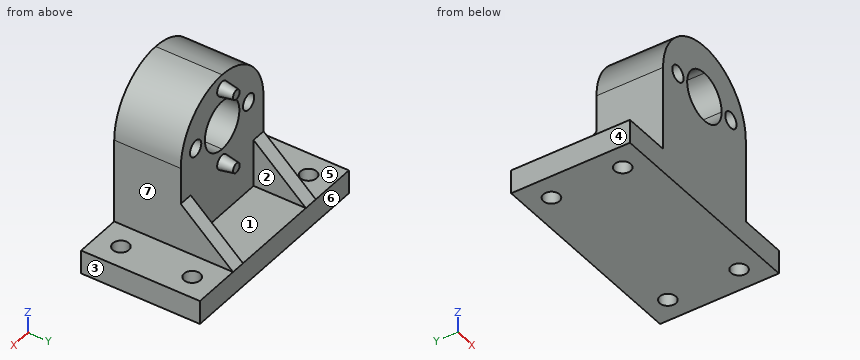
from build123d import *
from OCP.BRepFilletAPI import BRepFilletAPI_MakeChamfer

# Parameters (mm, degrees)
SKETCH1_R           = 1.7
BOSS_EXTRUDE1_DEPTH = 5
SKETCH2_R           = 1.7
BOSS_EXTRUDE2_DEPTH = 14
SKETCH3_R           = 1.5
BOSS_EXTRUDE3_DEPTH = 3
CHAMFER1_SIZE       = 3
CHAMFER1_SIZE_2     = 0.5
FILLET1_R           = 12.5
SKETCH4_W           = 3
SKETCH4_H           = 10
BOSS_EXTRUDE4_DEPTH = 11
CHAMFER2_SIZE       = 10
CHAMFER2_SIZE_2     = 11


with BuildPart() as part:
    # Sketch1 → Boss-Extrude1 (new body)
    with BuildSketch(Plane.XY):
        Polygon((-93.960167873, 235.92362241), (-129.123766163, 235.92362241), (-134.123766163, 235.92362241), (-134.123766163, 210.92362241), (-129.123766163, 210.92362241), (-93.960167873, 210.92362241), (-89.123766163, 210.92362241), (-89.123766163, 235.92362241), align=None)
        with Locations((-93.960167873, 215.92362241)):
            Circle(SKETCH1_R, mode=Mode.SUBTRACT)
        with Locations((-93.960167873, 230.92362241)):
            Circle(SKETCH1_R, mode=Mode.SUBTRACT)
        with Locations((-129.123766163, 215.92362241)):
            Circle(SKETCH1_R, mode=Mode.SUBTRACT)
        with Locations((-129.123766163, 230.92362241)):
            Circle(SKETCH1_R, mode=Mode.SUBTRACT)
    extrude(amount=BOSS_EXTRUDE1_DEPTH)

    # Sketch2 → Boss-Extrude2 (add)
    # profile 1 of 2: a face of its own
    with BuildSketch(Plane.XZ.offset(-210.92362241)):
        with BuildLine():
            Line((-111.623766166, 19.049999998), (-111.623766166, 5))
            Line((-111.623766166, 5), (-99.123766166, 5))
            Line((-99.123766166, 5), (-99.123766166, 35.249999998))
            Line((-99.123766166, 35.249999998), (-111.623766166, 35.249999998))
            Line((-111.623766166, 35.249999998), (-111.623766166, 29.449999998))
            ThreePointArc((-111.623766166, 29.449999998), (-107.946810904, 27.92695526), (-106.423766166, 24.249999998))
            ThreePointArc((-106.423766166, 24.249999998), (-107.946810904, 20.573044736), (-111.623766166, 19.049999998))
        make_face()
        with Locations(Location((-103.623766166, 24.249999998, 0), (0, 0, 270))):
            Circle(SKETCH2_R, mode=Mode.SUBTRACT)
    # profile 2 of 2: a face of its own
    with BuildSketch(Plane.XZ.offset(-210.92362241)):
        with BuildLine():
            Line((-124.123766166, 5), (-111.623766166, 5))
            Line((-111.623766166, 5), (-111.623766166, 19.049999998))
            ThreePointArc((-111.623766166, 19.049999998), (-116.823766166, 24.249999998), (-111.623766166, 29.449999998))
            Line((-111.623766166, 29.449999998), (-111.623766166, 35.249999998))
            Line((-111.623766166, 35.249999998), (-124.123766166, 35.249999998))
            Line((-124.123766166, 35.249999998), (-124.123766166, 5))
        make_face()
        with Locations(Location((-119.623766166, 24.249999998, 0), (0, 0, 270))):
            Circle(SKETCH2_R, mode=Mode.SUBTRACT)
    extrude(amount=-BOSS_EXTRUDE2_DEPTH)

    # Sketch3 → Boss-Extrude3 (add)
    with BuildSketch(Plane(origin=(0, 224.92362241, 0), x_dir=(1, 0, 0), z_dir=(0, 1, 0))):
        with Locations(Location((-111.623766166, -16.249999998, 0), (0, 0, 270))):
            Circle(SKETCH3_R)
        with Locations(Location((-111.623766166, -32.249999998, 0), (0, 0, 270))):
            Circle(SKETCH3_R)
    extrude(amount=BOSS_EXTRUDE3_DEPTH)

    # Chamfer1
    chamfer1_edges_1 = [part.edges().sort_by_distance(p)[0] for p in [
        (-111.623766166, 227.92362241, 14.749999998),
    ]]
    chamfer1_side_1 = [part.faces().sort_by_distance(p)[0] for p in [
        (-111.623766166, 227.91362241, 14.749999998),
    ]]
    chamfer1_edges_2 = [part.edges().sort_by_distance(p)[0] for p in [
        (-111.623766166, 227.92362241, 30.749999998),
    ]]
    chamfer1_side_2 = [part.faces().sort_by_distance(p)[0] for p in [
        (-111.623766166, 227.91362241, 30.749999998),
    ]]
    chamfer1 = BRepFilletAPI_MakeChamfer(part.part.solid().wrapped)
    for e in chamfer1_edges_1:
        chamfer1.Add(CHAMFER1_SIZE - 0.0001, CHAMFER1_SIZE_2 - 0.0001, e.wrapped, chamfer1_side_1[0].wrapped)
    for e in chamfer1_edges_2:
        chamfer1.Add(CHAMFER1_SIZE - 0.0001, CHAMFER1_SIZE_2 - 0.0001, e.wrapped, chamfer1_side_2[0].wrapped)
    add(Compound.cast(chamfer1.Shape()), mode=Mode.REPLACE)  # a hair under: the kernel refuses the full size

    # Fillet1
    fillet1_edges = [part.edges().sort_by_distance(p)[0] for p in [
        (-99.123766166, 217.92362241, 35.249999998),
        (-124.123766166, 217.92362241, 35.249999998),
    ]]
    fillet(fillet1_edges, radius=FILLET1_R - 0.0001)  # a hair under: the kernel refuses the full size

    # Sketch4 → Boss-Extrude4 (add)
    with BuildSketch(Plane(origin=(0, 224.92362241, 0), x_dir=(1, 0, 0), z_dir=(0, 1, 0))):
        with Locations((-122.623766166, -10)):
            Rectangle(SKETCH4_W, SKETCH4_H)
        with Locations((-100.623766166, -10)):
            Rectangle(SKETCH4_W, SKETCH4_H)
    extrude(amount=BOSS_EXTRUDE4_DEPTH)

    # Chamfer2
    chamfer2_edges_1 = [part.edges().sort_by_distance(p)[0] for p in [
        (-100.623766166, 235.92362241, 15),
    ]]
    chamfer2_side_1 = [part.faces().sort_by_distance(p)[0] for p in [
        (-100.623766166, 235.92362241, 14.8),
    ]]
    chamfer2_edges_2 = [part.edges().sort_by_distance(p)[0] for p in [
        (-122.623766166, 235.92362241, 15),
    ]]
    chamfer2_side_2 = [part.faces().sort_by_distance(p)[0] for p in [
        (-122.623766166, 235.92362241, 14.8),
    ]]
    chamfer2 = BRepFilletAPI_MakeChamfer(part.part.solid().wrapped)
    for e in chamfer2_edges_1:
        chamfer2.Add(CHAMFER2_SIZE - 0.0001, CHAMFER2_SIZE_2 - 0.0001, e.wrapped, chamfer2_side_1[0].wrapped)
    for e in chamfer2_edges_2:
        chamfer2.Add(CHAMFER2_SIZE - 0.0001, CHAMFER2_SIZE_2 - 0.0001, e.wrapped, chamfer2_side_2[0].wrapped)
    add(Compound.cast(chamfer2.Shape()), mode=Mode.REPLACE)  # a hair under: the kernel refuses the full size


solid = part.part
Read the model definition and answer for the solid it produces. Units are mm, in the model's axes. Face numbers are marked on the shaded views. A direction names the side the tool comes from. Round coordinates to 2 decimals unless told otherwise and drop trailing zeros. Loops run counter-clockwise (first coordinate to the right, second up) from the corner with the lowest first, then second, coordinate; pieces in that order, holes last. Notation, with made-up numbers: (28.5, 2) - (58.5, 2) arc R19 ccw to (58.5, 30) - close; hole circle Ø4 at (74.5, -12). An arc over 180 degrees is marked (long way). One line per question, with ' | ' between items. Start each with the question number.
Q1. Section B-B on y = 229.75 is taken. Give the vertices of the cut face in (x, z), plus the area to 3 significant figures.
Q2. Flat-ended cylindrical pins translate along their axes: pin 1 (3 mm diameter, centred on x = -128, y = 225, fed in from +Z); pin 2 (10 mm diameter, centred on x = -124.5, y = 222, fed in from +Z); pin 3 (11 mm diameter, centred on y = 230, z = 9, fed in from +X); pin 4 (0.6 mm diameter, centred on x = -112, z = 32.5, fed in from +Y). Find the tip coordinate at first contact, or state that the pin passes through.
Q3. For the marked faces 5, 6 and 7, determine the directions among +Z, -Z, +X, -X, +Y, -Y from which every point of the face is accessible in a straight line to the end or side of a thin tool.
Q4. Find the intervals of material crossed by L1, parallel to X at y = 228.25, z = 5.5; L2, parallel to X at y = 217, z = 24.25; L3, parallel to X at y = 212.75, z = 5.5, in increasing order.
Q5. For a pull along X with two mould halves and no side action, classify the marked faces 1, 2, 3 and 4 as +X half, -X half, draft (parallel to the pull), parting line (faces both ways), or undercut.
Q6. Section A-A on z = 23.5 is taken. Give the vertices of the cut face in (x, y), plus the area to 3 significant figures.
Q7. Section C-C on x = -118.5 is taken. Give the vertices of the cut face in (y, z), plus the area to 3 significant figures.
Established:
1) outline: (-134.12, 0) - (-130.35, 0) - (-130.35, 5) - (-134.12, 5) - close; (-127.89, 0) - (-95.19, 0) - (-95.19, 5) - (-99.12, 5) - (-99.12, 10.61) - (-102.12, 10.61) - (-102.12, 5) - (-121.12, 5) - (-121.12, 10.61) - (-124.12, 10.61) - (-124.12, 5) - (-127.89, 5) - close; (-92.73, 0) - (-89.12, 0) - (-89.12, 5) - (-92.73, 5) - close | area: 234 mm²
2) pin 1: z = 5 | pin 2: z = 32.46 | pin 3: x = -89.12 | pin 4: y = 227.92
3) face 5: +Z, -X, +Y, -Y | face 6: +Z, -Z, +X, -X, +Y | face 7: +Z, +X, +Y, -Y
4) L1: -124.12 to -121.12, -102.12 to -99.12 | L2: -124.03 to -121.32, -117.92 to -116.82, -106.42 to -105.32, -101.92 to -99.21 | L3: -124.12 to -99.12
5) face 1: undercut | face 2: undercut | face 3: +X half | face 4: -X half
6) outline: (-124.1, 210.92) - (-121.15, 210.92) - (-121.15, 224.92) - (-124.1, 224.92) - close; (-118.1, 210.92) - (-116.77, 210.92) - (-116.77, 224.92) - (-118.1, 224.92) - close; (-106.48, 210.92) - (-105.15, 210.92) - (-105.15, 224.92) - (-106.48, 224.92) - close; (-102.1, 210.92) - (-99.15, 210.92) - (-99.15, 224.92) - (-102.1, 224.92) - close | area: 120 mm²
7) outline: (210.92, 0) - (235.92, 0) - (235.92, 5) - (224.92, 5) - (224.92, 22.97) - (210.92, 22.97) - close; (210.92, 25.53) - (224.92, 25.53) - (224.92, 33.19) - (210.92, 33.19) - close | area: 484 mm²
